Build history of the part. All positions in model axes, mm. Face numbers are marked on the shaded views. A direction names the side the tool comes from. Give positions to 0.01 mm unless a question says otherwise; leave off trailing zeros. Order: outer loops, then holes, each group sorted by start corner. A loop starts at its lowest first (then second) coordinate and runs counter-clockwise, first axis right, second up. Notation, with made-up numbers: (-25.5, 73.25) - (-19.5, 73.25) arc R19 cw to (-19.5, 91.25) - close; hole circle Ø2 at (82.25, 35). An arc over 180 degrees is marked (long way). Use a Markdown table: item, result.
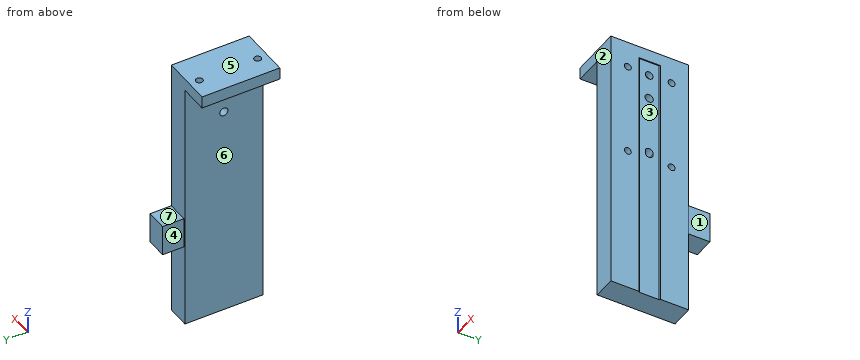
from build123d import *

# Parameters (mm, degrees)
BASE_EXTRUDE_DEPTH              = 5
BOSS_EXTRUDE1_DEPTH             = 105.5
BOSS_EXTRUDE3_DEPTH             = 5
F_3_4_DIAMETER_HOLE1_D          = 3.4
F_4_40_TAPPED_HOLE1_D           = 2.2606
F_4_40_TAPPED_HOLE1_DEPTH       = 7.239
F_4_40_TAPPED_HOLE1_CBORE_D     = 2.8448
F_4_40_TAPPED_HOLE1_CBORE_DEPTH = 4.064
F_4_40_TAPPED_HOLE1_TIP         = 0.679152758
F_4_40_TAPPED_HOLE2_D           = 2.2606
F_4_40_TAPPED_HOLE2_CBORE_D     = 2.8448
F_4_40_TAPPED_HOLE2_CBORE_DEPTH = 5.6896
CUT_EXTRUDE1_DEPTH              = 3.5
HOLE1_D                         = 3.1877
HOLE1_DEPTH                     = 2.54
SKETCH14_W                      = 8.53
SKETCH14_H                      = 12.7
BOSS_EXTRUDE2_DEPTH             = 8.73


with BuildPart() as part:
    # Sketch1 → Base-Extrude (new body)
    with BuildSketch(Plane.XY.offset(-942.568622791)):
        Polygon((-5.1213, 16), (15.9087, 16), (15.9087, 4.38), (15.5287, 4), (15.5287, -4), (15.9087, -4.38), (15.9087, -16), (-5.1213, -16), align=None)
    extrude(amount=BASE_EXTRUDE_DEPTH)

    # Sketch3 → Boss-Extrude1 (add)
    with BuildSketch(Plane(origin=(0, 0, -942.568622791), x_dir=(-1, 0, 0), z_dir=(0, 0, -1))):
        Polygon((-15.9087, 4.38), (-15.9087, 16), (-6.5913, 16), (-6.5913, -16), (-15.9087, -16), (-15.9087, -4.38), (-15.5287, -4), (-15.5287, 4), align=None)
    extrude(amount=BOSS_EXTRUDE1_DEPTH)

    # Sketch15 → Boss-Extrude3 (add)
    with BuildSketch(Plane.XY.offset(-937.568622791)):
        Polygon((15.9087, -4.38), (15.5287, -4), (15.5287, 4), (15.9087, 4.38), align=None)
    extrude(amount=-BOSS_EXTRUDE3_DEPTH)

    # 3.4 Diameter Hole1 (through all)
    with Locations(Plane(origin=(15.5287, 0, 0), x_dir=(0, 0, -1), z_dir=(1, 0, 0))):
        with Locations((958.868622791, 0)):
            Hole(F_3_4_DIAMETER_HOLE1_D / 2)

    # #4-40 Tapped Hole1
    with Locations(Plane(origin=(15.9087, 0, 0), x_dir=(0, 0, -1), z_dir=(1, 0, 0))):
        with Locations((948.568622791, 9), (986.568622791, 9), (948.568622791, -9), (986.568622791, -9)):
            CounterBoreHole(F_4_40_TAPPED_HOLE1_D / 2, F_4_40_TAPPED_HOLE1_CBORE_D / 2, F_4_40_TAPPED_HOLE1_CBORE_DEPTH, depth=F_4_40_TAPPED_HOLE1_DEPTH)
            with Locations((0, 0, -(F_4_40_TAPPED_HOLE1_DEPTH + F_4_40_TAPPED_HOLE1_TIP / 2))):  # 118° drill point
                Cone(0, F_4_40_TAPPED_HOLE1_D / 2, F_4_40_TAPPED_HOLE1_TIP, mode=Mode.SUBTRACT)

    # #4-40 Tapped Hole2 (through all)
    with Locations(Plane.XY.offset(-937.568622791)):
        with Locations((3.4087, 12), (3.4087, -12)):
            CounterBoreHole(F_4_40_TAPPED_HOLE2_D / 2, F_4_40_TAPPED_HOLE2_CBORE_D / 2, F_4_40_TAPPED_HOLE2_CBORE_DEPTH)

    # Sketch11 → Cut-Extrude1 (cut)
    with BuildSketch(Plane(origin=(15.5287, 0, 0), x_dir=(0, 0, -1), z_dir=(1, 0, 0))):
        with BuildLine():
            Line((983.162472791, 1.59385), (983.974772791, 1.59385))
            ThreePointArc((983.974772791, 1.59385), (985.568622791, 0), (983.974772791, -1.59385))
            Line((983.974772791, -1.59385), (983.162472791, -1.59385))
            ThreePointArc((983.162472791, -1.59385), (981.568622791, 0), (983.162472791, 1.59385))
        make_face()
    extrude(amount=-CUT_EXTRUDE1_DEPTH, mode=Mode.SUBTRACT)

    # Hole1
    with Locations(Plane(origin=(15.5287, 0, 0), x_dir=(0, 0, -1), z_dir=(1, 0, 0))):
        with Locations((948.568622791, 0)):
            Hole(HOLE1_D / 2, depth=HOLE1_DEPTH)

    # Sketch14 → Boss-Extrude2 (add)
    with BuildSketch(Plane(origin=(0, 16, 0), x_dir=(-1, 0, 0), z_dir=(0, 1, 0))):
        with Locations((-11.6337, -1007.418622791)):
            Rectangle(SKETCH14_W, SKETCH14_H)
    extrude(amount=BOSS_EXTRUDE2_DEPTH)


solid = part.part
1) Tool access for the marked faces 4, 5, 6 and 7: list every direction of +Z, -Z, +X, -X, +Y, -Y with a clear straight run to the whole face (end or side of a thin tool).
Computed:
| item | result |
|---|---|
| face 4 | +Z, -Z, -X, +Y |
| face 5 | +Z, +X, -X, +Y, -Y |
| face 6 | -Z, -X, +Y, -Y |
| face 7 | +Z, +X, -X, +Y |
2) Slice it at D-D (x = 1). Write the cut outline in (y, z).
Computed:
| item | result |
|---|---|
| outline | (-16, -942.57) - (16, -942.57) - (16, -937.57) - (-16, -937.57) - close |
3) Slice it at B-B (z = -975.5). Write the cut outline in (x, y).
Computed:
| item | result |
|---|---|
| outline | (6.59, -16) - (15.91, -16) - (15.91, -4.38) - (15.53, -4) - (15.53, 4) - (15.91, 4.38) - (15.91, 16) - (6.59, 16) - close |
4) Wall check: line 1 (Z direction, x = 9.4, y = -9); line 2 (Z direction, x = 9, y = 21.5); line 3 (Z direction, x = 9, y = 8). Give the ranges that are in metal, low to high. Write a range as from..to.
Computed:
| item | result |
|---|---|
| line 1 | z = -1048.07..-987.7, -985.44..-949.7, -947.44..-937.57 |
| line 2 | z = -1013.77..-1001.07 |
| line 3 | z = -1048.07..-987.1, -986.04..-949.1, -948.04..-937.57 |
5) Pin check, flat tips, straight feed: P1, Ø4, axis at y = 0, z = -948.57, coming from the +X side; P2, Ø8, axis at x = 7, z = -1021.5, coming from the +Y side; P3, Ø3.5, axis at x = 3.5, y = -5.5, coming from the -Z side. Stop position of each tip, or through.
Computed:
| item | result |
|---|---|
| P1 | stops at x = 15.53 |
| P2 | stops at y = 16 |
| P3 | stops at z = -942.57 |
6) Slice it at C-C (y = 0). Write the cut outline in (x, z), and give its area (3 significant figures).
Computed:
| item | result |
|---|---|
| outline | (-5.12, -942.57) - (6.59, -942.57) - (6.59, -957.17) - (15.53, -957.17) - (15.53, -950.16) - (12.99, -950.16) - (12.99, -946.97) - (15.53, -946.97) - (15.53, -942.57) - (15.91, -942.57) - (15.91, -937.57) - (-5.12, -937.57) - close; (6.59, -1048.07) - (15.53, -1048.07) - (15.53, -985.57) - (12.03, -985.57) - (12.03, -981.57) - (15.53, -981.57) - (15.53, -960.57) - (6.59, -960.57) - close |
| area | 996 mm² |
7) Two-plate mould, pull along Y, no slides. Class the marked faces 1, 2 and 3: +Y half, -Y half, draft (parallel to the pull), parting line (faces both ways), or undercut.
Computed:
| item | result |
|---|---|
| face 1 | draft |
| face 2 | -Y half |
| face 3 | undercut |
8) Slice it at A-A (y = 12). Write the cut outline in (x, z), and give its area (3 significant figures).
Computed:
| item | result |
|---|---|
| outline | (-5.12, -942.57) - (1.99, -942.57) - (1.99, -937.57) - (-5.12, -937.57) - close; (4.83, -942.57) - (6.59, -942.57) - (6.59, -1048.07) - (15.91, -1048.07) - (15.91, -937.57) - (4.83, -937.57) - close |
| area | 1,070 mm² |
